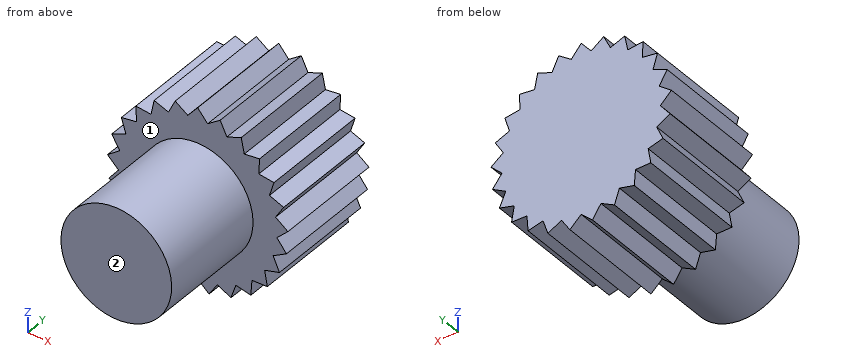
from build123d import *

# Parameters (mm, degrees)
SKETCH1_R           = 1.5
BOSS_EXTRUDE1_DEPTH = 3.01
BOSS_EXTRUDE2_DEPTH = 3


with BuildPart() as part:
    # Sketch1 → Boss-Extrude1 (new body)
    with BuildSketch(Plane(origin=(0, 0, 0), x_dir=(1, 0, 0), z_dir=(0, 1, 0))):
        with Locations(Location((0, 0, 0), (0, 0, 270))):
            Circle(SKETCH1_R)
    extrude(amount=BOSS_EXTRUDE1_DEPTH)

    # Sketch2 → Boss-Extrude2 (add)
    with BuildSketch(Plane(origin=(0, 3.01, 0), x_dir=(1, 0, 0), z_dir=(0, 1, 0))):
        Polygon((0.307066422, 2.430681018), (0.534683257, 2.082453796), (0.901905154, 2.27795239), (1.035770399, 1.884059362), (1.440073868, 1.982091636), (1.471776278, 1.567282549), (1.887757445, 1.561688775), (1.81530504, 1.152027609), (2.216826279, 1.043159264), (2.04477151, 0.664386538), (2.406603764, 0.459084221), (2.145757466, 0.134999617), (2.445165485, -0.153836773), (2.111917589, -0.402869826), (2.330088465, -0.757091636), (1.945378163, -0.915425477), (2.068603417, -1.312775648), (1.656603472, -1.370461578), (1.67714041, -1.785973137), (1.263738292, -1.739386538), (1.180296502, -2.146951366), (0.791467788, -1.999019445), (0.609290224, -2.373028745), (0.269466452, -2.133046608), (0, -2.45), (-0.269466452, -2.133046608), (-0.609290224, -2.373028745), (-0.791467788, -1.999019445), (-1.180296502, -2.146951366), (-1.263738292, -1.739386538), (-1.67714041, -1.785973137), (-1.656603472, -1.370461578), (-2.068603417, -1.312775648), (-1.945378163, -0.915425477), (-2.330088465, -0.757091636), (-2.111917589, -0.402869826), (-2.445165485, -0.153836773), (-2.145757466, 0.134999617), (-2.406603764, 0.459084221), (-2.04477151, 0.664386538), (-2.216826279, 1.043159264), (-1.81530504, 1.152027609), (-1.887757445, 1.561688775), (-1.471776278, 1.567282549), (-1.440073868, 1.982091636), (-1.035770399, 1.884059362), (-0.901905154, 2.27795239), (-0.534683257, 2.082453796), (-0.307066422, 2.430681018), (0, 2.15), align=None)
    extrude(amount=BOSS_EXTRUDE2_DEPTH)


solid = part.part
Design review of the part built by this model. Coordinates are the model's own, in mm. Face numbers are marked on the shaded views. A direction names the side the tool comes from. Give positions to 0.01 mm unless a question says otherwise; leave off trailing zeros. Loops run counter-clockwise (first coordinate to the right, second up) from the corner with the lowest first, then second, coordinate; pieces in that order, holes last. Notation, with made-up numbers: (78, 89) -> (120, 89) arc R17 cw to (120, 117) -> close; hole circle Ø9 at (80, -2). An arc over 180 degrees is marked (long way). One line per question, with ' | ' between items. Start each with the question number.
(1) We need section A-A (x = -0.45). State the section outline as (y, z) points, and give its area (3 significant figures).
(2) For line 1 (X direction, y = 2.5, z = -0.3); line 2 (Y direction, x = 1.25, z = -1.35); line 3 (X direction, y = 4.25, z = 1.4), list the stretches that pass through material, from the lowest coordinate up.
(3) We need section C-C (z = 0.5). State the section outline as (x, y) points.
(4) For the marked faces 1 and 2, list the 3-axis set-ups (+Z, -Z, +X, -X, +Y, -Y) from which the entire face can be reached by the end or side of a thin tool; tool diameter is ignored.
(5) Insertion check: P1, Ø1.5, axis at y = 3.5, z = -1, coming from the +X side; P2, Ø1, axis at x = 1, y = 4, coming from the +Z side; P3, Ø2, axis at y = 4, z = 0, coming from the -X side. Each pin has a flat end and moves straight along its axis. Give the tip position at first contact, or say it passes through.
(6) We need section B-B (y = 2.25). State the section outline as (x, z) points.
The answers:
1) outline: (0, -1.43) -> (3.01, -1.43) -> (3.01, -2.21) -> (6.01, -2.21) -> (6.01, 2.26) -> (3.01, 2.26) -> (3.01, 1.43) -> (0, 1.43) -> close | area: 22.0 mm^2
2) line 1: x = -1.47 to 1.47 | line 2: y = 3.01 to 6.01 | line 3: x = -1.66 to 1.66
3) outline: (-2.17, 3.01) -> (-1.41, 3.01) -> (-1.41, 0) -> (1.41, 0) -> (1.41, 3.01) -> (2.17, 3.01) -> (2.17, 6.01) -> (-2.17, 6.01) -> close
4) face 1: -Y | face 2: +Z, -Z, +X, -X, -Y
5) P1: stops at x = 2.41 | P2: stops at z = 2.37 | P3: stops at x = -2.45
6) outline: circle Ø3 at (0, 0)
